```python
from build123d import *

# Parameters (mm, degrees)
EXTRUDE_1219_DEPTH     = 7.95
CUT_EXTRUDE_1748_DEPTH = 86.222223289
FILLET_1_R             = 1
CUT_EXTRUDE_3045_DEPTH = 86.222223289
FILLET_START           = -9
FILLET_2_DEPTH         = 10
FILLET_3_DEPTH         = 10


with BuildPart() as part:
    # Эскиз1 → Extrude 1219 (new body)
    with BuildSketch(Plane.XY):
        with BuildLine():
            Line((-59.003125249, 0), (-59.003125249, 7.5))
            Line((-59.003125249, 7.5), (-67.003125249, 7.5))
            ThreePointArc((-67.003125249, 7.5), (-75.989225627, 4.93086969), (-82.259271551, -2))
            Line((-82.259271551, -2), (-84.259271551, -2))
            ThreePointArc((-84.259271551, -2), (-78.132206164, 6.673633304), (-68.047161318, 10))
            Line((-68.047161318, 10), (0, 10))
            Line((0, 10), (22.496874751, 10))
            ThreePointArc((22.496874751, 10), (31.915339808, 6.61174951), (37.016858777, -2))
            Line((37.016858777, -2), (35.016858777, -2))
            ThreePointArc((35.016858777, -2), (30.354991574, 4.856157589), (22.496874751, 7.5))
            Line((22.496874751, 7.5), (20.996874751, 7.5))
            Line((20.996874751, 7.5), (20.996874751, 0))
            ThreePointArc((20.996874751, 0), (-19.003125249, 5.431677052), (-59.003125249, 0))
        make_face()
    extrude(amount=-EXTRUDE_1219_DEPTH)

    # Эскиз4 → Cut-Extrude 1748 (cut, through all)
    with BuildSketch(Plane.XY):
        with BuildLine():
            Line((-56.503125249, 2.5), (-51.503125249, 2.5))
            ThreePointArc((-51.503125249, 2.5), (-50.503125249, 1.5), (-51.503125249, 0.5))
            Line((-51.503125249, 0.5), (-56.503125249, 0.5))
            ThreePointArc((-56.503125249, 0.5), (-57.503125249, 1.5), (-56.503125249, 2.5))
        make_face()
        with BuildLine():
            Line((13.496874751, 2.5), (18.496874751, 2.5))
            ThreePointArc((18.496874751, 2.5), (19.496874751, 1.5), (18.496874751, 0.5))
            Line((18.496874751, 0.5), (13.496874751, 0.5))
            ThreePointArc((13.496874751, 0.5), (12.496874751, 1.5), (13.496874751, 2.5))
        make_face()
    extrude(amount=-CUT_EXTRUDE_1748_DEPTH, mode=Mode.SUBTRACT)

    # Скругление1
    # the kernel refuses this fillet: 1 mm, written as the material it adds along each edge
    with BuildSketch(Plane(origin=(20.996874751, 7.5, 0), x_dir=(0, -1, 0), z_dir=(0, 0, -1))) as fillet_1_piece_1:
        with BuildLine():
            CenterArc((FILLET_1_R, -FILLET_1_R), FILLET_1_R, 90, 90)
            Line((0, -FILLET_1_R), (0, 0))
            Line((0, 0), (FILLET_1_R, 0))
        make_face()
    extrude(amount=7.95)
    with BuildSketch(Plane(origin=(-59.003125249, 7.5, 0), x_dir=(0, -1, 0), z_dir=(0, 0, -1))) as fillet_1_piece_2:
        with BuildLine():
            CenterArc((FILLET_1_R, FILLET_1_R), FILLET_1_R, 180, 90)
            Line((0, FILLET_1_R), (0, 0))
            Line((0, 0), (FILLET_1_R, 0))
        make_face()
    extrude(amount=7.95)
    # the kernel refuses this fillet: 1 mm, written as the material it takes off along each edge
    with BuildSketch(Plane(origin=(20.996874751, 0, 3.270843206), x_dir=(-0.9649388241572373, 0.26247488572061173, 0), z_dir=(0, 0, -1))) as fillet_1_2_piece_1:
        with BuildLine():
            CenterArc((1.308344503, 0.999990553), FILLET_1_R, 164.783036074, 104.967917899)
            Line((0.343405679, 1.262465439), (0, 0))
            ThreePointArc((0, 0), (0.651998922, 0.001417015), (1.303997843, 0))
        make_face()
    extrude(amount=14.491686412, mode=Mode.SUBTRACT)
    with BuildSketch(Plane(origin=(-59.003125249, 0, 3.270843206), x_dir=(0, 1, 0), z_dir=(0, 0, -1))) as fillet_1_2_piece_2:
        with BuildLine():
            CenterArc((1.308337282, 1), FILLET_1_R, 165.032082101, 104.967917899)
            ThreePointArc((0.342266685, 1.258278146), (0.172500676, 0.628767142), (0, 0))
            Line((0, 0), (1.308337282, 0))
        make_face()
    extrude(amount=14.491686412, mode=Mode.SUBTRACT)
    with BuildSketch(Plane(origin=(18.869217353, 0.571904645, -11.41789989), x_dir=(0.6247425525309795, 0.7808308030918583, 0), z_dir=(0, 0, 1))) as fillet_1_2_piece_3:
        with BuildLine():
            CenterArc((1.476201521, -0.870557233), FILLET_1_R, 119.476541698, 84.032444608)
            ThreePointArc((0.559203998, -1.26945013), (0.281069449, -0.63407864), (0, 0))
            ThreePointArc((0, 0), (0.492067174, -0.129442767), (0.984134348, 0))
        make_face()
    extrude(amount=14.88579978, mode=Mode.SUBTRACT)
    with BuildSketch(Plane(origin=(-56.87546785, 0.571904645, -11.41789989), x_dir=(-0.9664237291257997, -0.2569536452019758, 0), z_dir=(0, 0, 1))) as fillet_1_2_piece_4:
        with BuildLine():
            CenterArc((1.391783822, -0.99998931), FILLET_1_R, 90.264928981, 84.032444608)
            ThreePointArc((0.396732806, -0.900623947), (0.316825083, -0.398129879), (0, 0))
            ThreePointArc((0, 0), (0.693579978, -0.001603519), (1.387159956, 0))
        make_face()
    extrude(amount=14.88579978, mode=Mode.SUBTRACT)

    # Эскиз3 → Cut-Extrude 3045 (cut, through all)
    with BuildSketch(Plane.XY):
        with BuildLine():
            Line((-28.348469228, 10), (-13.651530772, 10))
            ThreePointArc((-13.651530772, 10), (-21, 8), (-28.348469228, 10))
        make_face()
    extrude(amount=-CUT_EXTRUDE_3045_DEPTH, mode=Mode.SUBTRACT)

    # Скругление2: read off the stored shape, not the designer's step
    # Скругление2 outline → Скругление2 (cut)
    with BuildSketch(Plane.XY.offset(FILLET_START)):
        with BuildLine():
            add(Edge.make_bspline(
                [(-82.863119301, -2), (-82.449925955, -1.99999996), (-82.147973363, -1.770582651), (-81.991237502, -1.477750248)],
                knots=[0.617138018, 0.617138018, 0.617138018, 0.617138018, 1, 1, 1, 1], degree=3, weights=[0.553450152, 0.609956112, 0.758806062, 1]))
            Line((-82.863119301, -2), (-82.259271551, -2))
            ThreePointArc((-82.259271551, -2), (-82.127508876, -1.737718125), (-81.991237502, -1.477750248))
        make_face()
        with BuildLine():
            add(Edge.make_bspline(
                [(-83.781008367, -0.643067451), (-84.028353334, -1.25998415), (-83.741746006, -2.000000086), (-82.863119301, -2)],
                knots=[0, 0, 0, 0, 0.617138018, 0.617138018, 0.617138018, 0.617138018], degree=3, weights=[1, 0.611217733, 0.462367784, 0.553450152]))
            ThreePointArc((-83.781008367, -0.643067451), (-84.03454269, -1.316457352), (-84.259271551, -2))
            Line((-84.259271551, -2), (-82.863119301, -2))
        make_face()
    extrude(amount=FILLET_2_DEPTH, mode=Mode.SUBTRACT)

    # Скругление3: read off the stored shape, not the designer's step
    # Скругление3 outline → Скругление3 (cut)
    with BuildSketch(Plane.XY.offset(FILLET_START)):
        with BuildLine():
            add(Edge.make_bspline(
                [(35.753175475, -2), (36.580087454, -2.000000006), (36.88300902, -1.319995015), (36.713739215, -0.726922424)],
                knots=[0.42186979, 0.42186979, 0.42186979, 0.42186979, 1, 1, 1, 1], degree=3, weights=[0.524198025, 0.465452398, 0.624053056, 1]))
            Line((35.753175475, -2), (37.016858777, -2))
            ThreePointArc((37.016858777, -2), (36.879391808, -1.360105716), (36.713739215, -0.726922424))
        make_face()
        with BuildLine():
            add(Edge.make_bspline(
                [(34.80724517, -1.32210817), (34.931629097, -1.688611726), (35.257891746, -1.999999996), (35.753175475, -2)],
                knots=[0, 0, 0, 0, 0.42186979, 0.42186979, 0.42186979, 0.42186979], degree=3, weights=[1, 0.725666199, 0.567065541, 0.524198025]))
            ThreePointArc((34.80724517, -1.32210817), (34.916677882, -1.65962369), (35.016858777, -2))
            Line((35.016858777, -2), (35.753175475, -2))
        make_face()
    extrude(amount=FILLET_3_DEPTH, mode=Mode.SUBTRACT)


solid = part.part
```
Design review of the part built by this model. Coordinates are the model's own, in mm. A direction names the side the tool comes from. Coordinates: 2 decimals unless noted, no trailing zeros. Order: outer loops, then holes, each group sorted by start corner. A loop starts at its lowest first (then second) coordinate and runs counter-clockwise, first axis right, second up.
1) For faces 1 (the flat face through (20.997, 4, -4)), 2 (the cylindrical face through (-77.66, 7.01, -3.92)), list the 3-axis set-ups (+Z, -Z, +X, -X, +Y, -Y) from which the entire face can be reached by the end or side of a thin tool; tool diameter is ignored.
2) Take a section at B-B, the plane x = -3. Give the boundary of the cut face in (y, z), and give its area (3 significant figures).
3) Wall thickness on line 1 along X through (y, z) = (1.5, -3.5); line 2 along X through (y, z) = (5.75, -7); line 3 along Y through (x, z) = (-54, -4.25): over which ranges is each line inside the solid? List them lowest first.
4) Clearance check with flat-ended pins moving along their axes: pin 1 (1.6 mm diameter, centred on y = 2.5, z = -2.5, fed in from -X); pin 2 (4 mm diameter, centred on y = 8, z = -3, fed in from -X); pin 3 (1 mm diameter, centred on x = 8, y = 8, fed in from +Z); pin 4 (1.5 mm diameter, centred on x = 15, z = -4, fed in from -Y). State where each tip first meets the part, or that it passes through.
5) Take a section at A-A, the plane x = -54. Give the boundary of the cut face in (y, z).
Returned:
1. face 1: +Z, -Z, -Y
1. face 2: +Z, -Z, -X, +Y
2. outline: (4.58, -7.95) - (10, -7.95) - (10, 0) - (4.58, 0) - close
2. area: 43.1 mm2
3. line 1: x = -82.74 to -79.96, -59 to -57.5, 19.5 to 21, 33.45 to 35.88
3. line 2: x = -79.27 to -74.52, -59 to 21, 29.01 to 32.87
3. line 3: y = 2.5 to 10
4. pin 1: stops at x = -82.62
4. pin 2: stops at x = -78.98
4. pin 3: stops at z = 0
4. pin 4: stops at y = 2.5
5. outline: (2.5, -7.95) - (10, -7.95) - (10, 0) - (2.5, 0) - close
